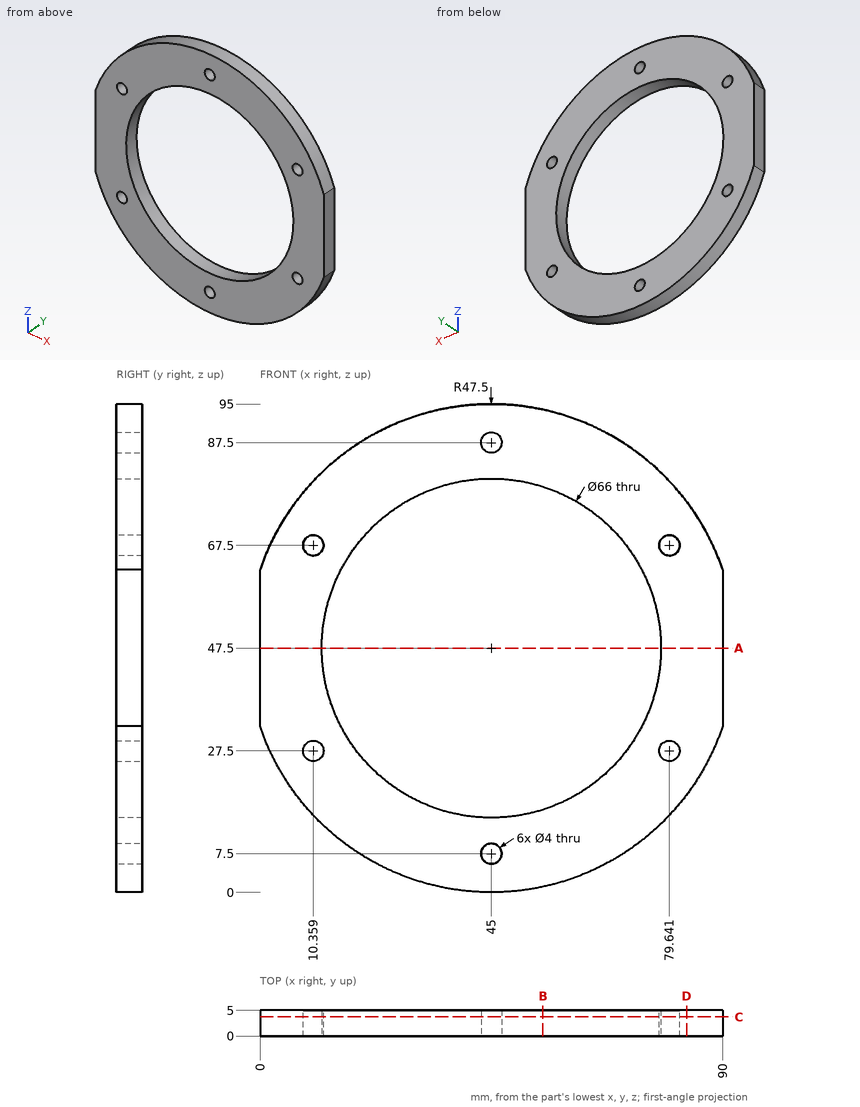
Study the drawing (mm; zero at the part's minimum x, y, z) and answer. Coordinates: 2 decimals unless noted, no trailing zeros. Write each loop counter-clockwise with the first axis right and the second up, starting at its lowest first coordinate (ties: lowest second). Pieces come first, ordered by that corner, then holes. Notation, with made-up numbers: (3, -30.75) - (37, -30.75) arc R13 cw to (37, -18.75) - close; hole circle Ø7 at (53, -25). An arc over 180 degrees is marked (long way). Return JSON: item names as keys, results as strings. Group by question number.
1. Straight lines are drawn through the part: L1, parallel to X at y = 3.95, z = 47.5; L2, parallel to X at y = 1.75, z = 27.5; L3, parallel to Z at x = 43.5, y = 1.5. For each, find the intervals that lie inside material, in ascending order.
2. A cutting plane is placed at C-C, the plane y = 3.7. Determine the outline of the cut face in (x, z), plus the area to 3 significant figures.
3. Given pin 1 (12 mm diameter, centred on x = 20.5, z = 33.5, fed in from -Y), flat-ended and moving along its own axis, determine where the tip first touches the part or whether it passes through.
4. A cutting plane is placed at B-B, the plane x = 55. Determine the outline of the cut face in (y, z), plus the area to 3 significant figures.
5. A cutting plane is placed at D-D, the plane x = 83. Determine the outline of the cut face in (y, z).
6. A cutting plane is placed at A-A, the plane z = 47.5. Determine the outline of the cut face in (x, y).
Ans:
{
 "1": {"L1": "0 to 12, 78 to 90", "L2": "1.92 to 8.36, 12.36 to 18.75, 71.25 to 77.64, 81.64 to 88.08", "L3": "0.02 to 6.18, 8.82 to 14.53, 80.47 to 86.18, 88.82 to 94.98"},
 "2": {"outline": "(0, 32.29) arc R47.5 ccw to (90, 32.29) - (90, 62.71) arc R47.5 ccw to (0, 62.71) - close; hole circle Ø4 at (10.36, 27.5); hole circle Ø4 at (10.36, 67.5); hole circle Ø66 at (45, 47.5); hole circle Ø4 at (45, 7.5); hole circle Ø4 at (45, 87.5); hole circle Ø4 at (79.64, 27.5); hole circle Ø4 at (79.64, 67.5)", "area": "3,490 mm²"},
 "3": {"pin 1": "y = 0"},
 "4": {"outline": "(0, 1.06) - (5, 1.06) - (5, 16.05) - (0, 16.05) - close; (0, 78.95) - (5, 78.95) - (5, 93.94) - (0, 93.94) - close", "area": "150 mm²"},
 "5": {"outline": "(0, 19) - (5, 19) - (5, 76) - (0, 76) - close"},
 "6": {"outline": "(0, 0) - (12, 0) - (12, 5) - (0, 5) - close; (78, 0) - (90, 0) - (90, 5) - (78, 5) - close"}
}
